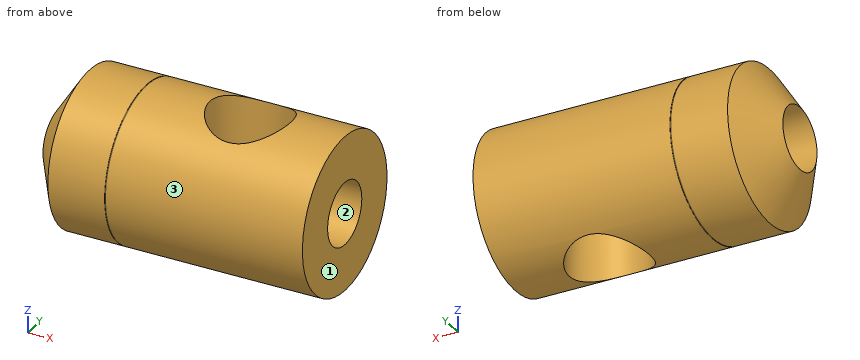
from build123d import *

# Parameters (mm, degrees)
SKETCH2_R               = 4.9276
CUT_EXTRUDE1_DEPTH      = 10.42975
CUT_EXTRUDE1_DEPTH_BACK = 10.42975


with BuildPart() as part:
    # Sketch1 → Revolve1 (revolve)
    with BuildSketch(Plane.XY):
        Polygon((-1.7145, 3.81), (15.6845, 3.81), (15.6845, 9.42975), (-8.3947, 9.42975), (-8.3947, 9.398), (-8.4455, 9.398), (-8.4963, 9.398), (-8.4963, 9.42975), (-15.4305, 9.42975), (-19.1135, 3.81), align=None)
    revolve(axis=Axis((0, 0, 0), (-1, 0, 0)))

    # Sketch2 → Cut-Extrude1 (cut, two sides)
    with BuildSketch(Plane.XY) as cut_extrude1_sk:
        with Locations((4.1529, 0)):
            Circle(SKETCH2_R)
    extrude(amount=CUT_EXTRUDE1_DEPTH, mode=Mode.SUBTRACT)
    extrude(cut_extrude1_sk.sketch, amount=-CUT_EXTRUDE1_DEPTH_BACK, mode=Mode.SUBTRACT)


solid = part.part
Geometry check sheet. Reference: the model listing, model coordinates, mm. Face numbers are marked on the shaded views. Round coordinates to 2 decimals unless told otherwise and drop trailing zeros. Order: outer loops, then holes, each group sorted by start corner. A loop starts at its lowest first (then second) coordinate and runs counter-clockwise, first axis right, second up. Notation, with made-up numbers: M 51.25,-28 L 109.25,-28 A14 cw 109.25,-11 Z; hole C 66,-3.5 d3. An arc over 180 degrees is marked long. Write each question's results on one line, items separated by ' | '. Start each with the question number.
1. Draft check along Y on the marked faces 1, 2 and 3. Enter one of: pulls with the +Y half, pulls with the -Y half, needs draft (parallel to the pull), parting line crosses it, or undercut.
2. Material ranges on L1, parallel to Z at x = -14, y = 0; L2, parallel to X at y = 3.25, z = -3, recorded low to high. Write a range as from..to.
3. Go/stop test with flat-tipped pins: P1, Ø2, axis at x = 3.5, y = -2.5, coming from the -Z side; P2, Ø1.5, axis at x = 8, y = 2, coming from the +Z side; P3, Ø1.5, axis at y = -1.5, z = -6.5, coming from the -X side; P4, Ø2, axis at x = 0, z = 6, coming from the -Y side (3 decimals). Record where each tip stops, or that it passes through.
4. Cross-section at A-A on y = 0. Give the number of separate pieces and of enclosed holes in the cut face, plus the area to 3 significant figures.
5. Cross-section at B-B on x = -5. Record the boundary of the cut face in (y, z), plus the area to 3 significant figures.
6. Cross-section at C-C on x = -16.5. Record the boundary of the cut face in (y, z), plus the area to 3 significant figures.
Resolved:
1) face 1: needs draft | face 2: undercut | face 3: parting line crosses it
2) L1: -9.43..-3.81, 3.81..9.43 | L2: -18.71..0.45, 7.86..15.68
3) P1: through | P2: z = 9.25 | P3: x = -17.73 | P4: y = -7.995
4) separate pieces: 4 | enclosed holes: 0 | area: 260 mm2
5) outline: C 0,0 d18.86; hole C 0,0 d7.62 | area: 234 mm2
6) outline: C 0,0 d15.6; hole C 0,0 d7.62 | area: 145 mm2
